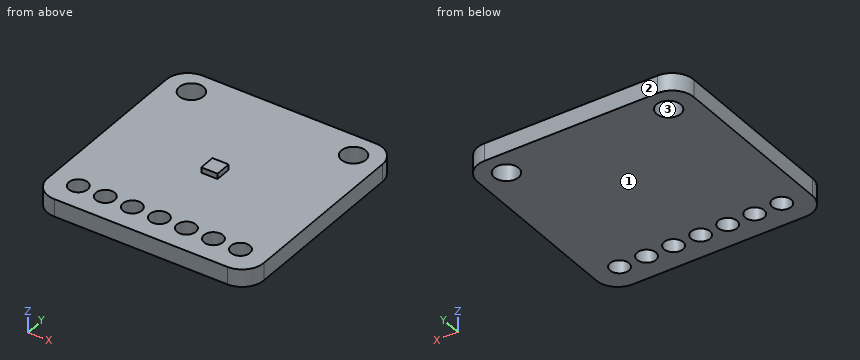
```python
from build123d import *

# Parameters (mm, degrees)
SKETCH1_R           = 1.143
SKETCH1_R_2         = 0.889
BOSS_EXTRUDE1_DEPTH = 1.651
SKETCH2_W           = 1.524
SKETCH2_H           = 1.524
BOSS_EXTRUDE2_DEPTH = 0.508


with BuildPart() as part:
    # Sketch1 → Boss-Extrude1 (new body)
    with BuildSketch(Plane.XY):
        with BuildLine():
            Line((-8.057940151, 8.672775064), (8.198059849, 8.672775064))
            ThreePointArc((8.198059849, 8.672775064), (9.634900828, 8.077616044), (10.230059849, 6.640775064))
            Line((10.230059849, 6.640775064), (10.230059849, -9.615224936))
            ThreePointArc((10.230059849, -9.615224936), (9.634900828, -11.052065915), (8.198059849, -11.647224936))
            Line((8.198059849, -11.647224936), (-8.057940151, -11.647224936))
            ThreePointArc((-8.057940151, -11.647224936), (-9.49478113, -11.052065915), (-10.089940151, -9.615224936))
            Line((-10.089940151, -9.615224936), (-10.089940151, 6.640775064))
            ThreePointArc((-10.089940151, 6.640775064), (-9.49478113, 8.077616044), (-8.057940151, 8.672775064))
        make_face()
        with Locations(Location((-7.549940151, 6.386775064, 0), (0, 0, 180))):
            Circle(SKETCH1_R, mode=Mode.SUBTRACT)
        with Locations(Location((7.690059849, 6.386775064, 0), (0, 0, 180))):
            Circle(SKETCH1_R, mode=Mode.SUBTRACT)
        with Locations(Location((0.070059849, -9.107224936, 0), (0, 0, 180))):
            Circle(SKETCH1_R_2, mode=Mode.SUBTRACT)
        with Locations(Location((2.610059849, -9.107224936, 0), (0, 0, 180))):
            Circle(SKETCH1_R_2, mode=Mode.SUBTRACT)
        with Locations(Location((5.150059849, -9.107224936, 0), (0, 0, 180))):
            Circle(SKETCH1_R_2, mode=Mode.SUBTRACT)
        with Locations(Location((7.690059849, -9.107224936, 0), (0, 0, 180))):
            Circle(SKETCH1_R_2, mode=Mode.SUBTRACT)
        with Locations(Location((-2.469940151, -9.107224936, 0), (0, 0, 180))):
            Circle(SKETCH1_R_2, mode=Mode.SUBTRACT)
        with Locations(Location((-5.009940151, -9.107224936, 0), (0, 0, 180))):
            Circle(SKETCH1_R_2, mode=Mode.SUBTRACT)
        with Locations(Location((-7.549940151, -9.107224936, 0), (0, 0, 180))):
            Circle(SKETCH1_R_2, mode=Mode.SUBTRACT)
    extrude(amount=BOSS_EXTRUDE1_DEPTH)

    # Sketch2 → Boss-Extrude2 (add)
    with BuildSketch(Plane.XY.offset(1.651)):
        with Locations((0.070059849, -1.487224936)):
            Rectangle(SKETCH2_W, SKETCH2_H)
    extrude(amount=BOSS_EXTRUDE2_DEPTH)


solid = part.part
```
Could you check a few things on this model? Use its own coordinates, in mm. Face numbers are marked on the shaded views. Give positions to 0.01 mm unless a question says otherwise; leave off trailing zeros. Loops run counter-clockwise (first coordinate to the right, second up) from the corner with the lowest first, then second, coordinate; pieces in that order, holes last. Notation, with made-up numbers: (68, -5.5) - (126, -5.5) arc R20 ccw to (126, 14.5) - close; hole circle Ø4 at (77, 26). An arc over 180 degrees is marked (long way). Answer in a Markdown table with one row per item. Add a question column.
Q1. We'd pull the mould along Y, two halves only. Please class the marked faces 1, 2 and 3: +Y half, -Y half, draft (parallel to the pull), parting line (faces both ways), or undercut.
Q2. If we section it at C-C (x = -7): List the corners of the cut face in (y, z) for me, plus the area to 3 significant figures.
Q3. For pin 1 (0.6 mm diameter, centred on x = 0, z = 2, fed in from +Y); pin 2 (8 mm diameter, centred on x = -2, y = -3, fed in from -Z); pin 3 (0.6 mm diameter, centred on y = -1.5, z = 2, fed in from +X); pin 4 (2.5 mm diameter, centred on x = 7.69, y = 6.39, fed in from +Z), each with a flat end and sliding along its axis, tell me the tip position at first contact or that it passes through.
Q4. If we section it at D-D (z = 1.25): State how many separate pieces and enclosed holes the cut face has, plus the area to 3 significant figures.
Q5. If we section it at B-B (y = -1): List the corners of the cut face in (x, z) for me.
Q6. Please list where these lines run through material, in increasing order: L1, parallel to X at y = 6.5, z = 1.05; L2, parallel to X at y = 5.75, z = 1.1; L3, parallel to Y at x = -5, z = 0.2. Write a range as from..to.
Q7. If we section it at A-A (x = 2): List the corners of the cut face in (y, z) for me.
The answers:
| question | item | result |
|---|---|---|
| 1 | face 1 | draft |
| 1 | face 2 | +Y half |
| 1 | face 3 | undercut |
| 2 | outline | (-11.65, 0) - (-9.81, 0) - (-9.81, 1.65) - (-11.65, 1.65) - close; (-8.41, 0) - (5.38, 0) - (5.38, 1.65) - (-8.41, 1.65) - close; (7.39, 0) - (8.67, 0) - (8.67, 1.65) - (7.39, 1.65) - close |
| 2 | area | 27.9 mm^2 |
| 3 | pin 1 | stops at y = -0.73 |
| 3 | pin 2 | stops at z = 0 |
| 3 | pin 3 | stops at x = 0.83 |
| 3 | pin 4 | stops at z = 1.65 |
| 4 | separate pieces | 1 |
| 4 | enclosed holes | 9 |
| 4 | area | 384 mm^2 |
| 5 | outline | (-10.09, 0) - (10.23, 0) - (10.23, 1.65) - (0.83, 1.65) - (0.83, 2.16) - (-0.69, 2.16) - (-0.69, 1.65) - (-10.09, 1.65) - close |
| 6 | L1 | x = -10.09..-8.69, -6.41..6.55, 8.83..10.23 |
| 6 | L2 | x = -10.09..-8.5, -6.6..6.74, 8.64..10.23 |
| 6 | L3 | y = -11.65..-10, -8.22..8.67 |
| 7 | outline | (-11.65, 0) - (-9.75, 0) - (-9.75, 1.65) - (-11.65, 1.65) - close; (-8.46, 0) - (8.67, 0) - (8.67, 1.65) - (-8.46, 1.65) - close |
